from build123d import *

# Parameters (mm, degrees)
F0_W     = 70.4432
F0_H     = 95.6654
F0_R     = 27.5
F1_DEPTH = 25
F2_R     = 5.08


with BuildPart() as f1:
    # F0 (on Top) → F1 (new body)
    with BuildSketch(Plane.XY):
        with Locations((0, -15.2273)):
            Rectangle(F0_W, F0_H)
        Circle(F0_R, mode=Mode.SUBTRACT)
    extrude(amount=F1_DEPTH)

    # F2
    f2_edges = [f1.edges().sort_by_distance(p)[0] for p in [
        (35.2216, -15.2273, 25),
        (35.2216, -15.2273, 0),
        (-35.2216, -15.2273, 25),
        (-35.2216, -15.2273, 0),
        (-35.2216, 32.6054, 12.5),
        (35.2216, 32.6054, 12.5),
        (0, 32.6054, 25),
        (0, 32.6054, 0),
    ]]
    fillet(f2_edges, radius=F2_R)


solid = f1.part
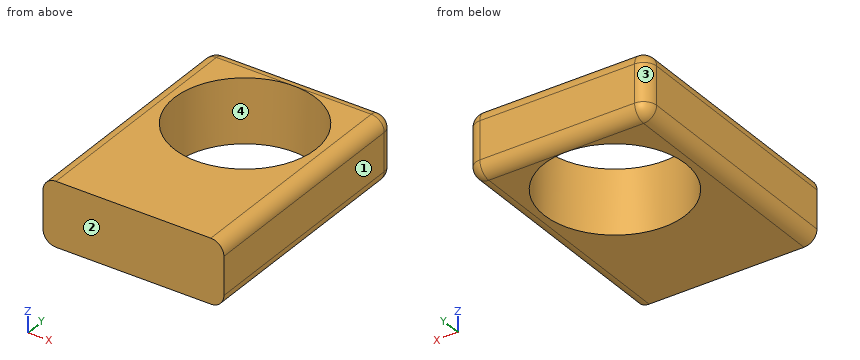
Geometry check sheet. Reference: the model listing, model coordinates, mm. Face numbers are marked on the shaded views. Round coordinates to 2 decimals unless told otherwise and drop trailing zeros. Order: outer loops, then holes, each group sorted by start corner. A loop starts at its lowest first (then second) coordinate and runs counter-clockwise, first axis right, second up. Notation, with made-up numbers: (14.25, -34.5) - (45.25, -34.5) arc R23 ccw to (45.25, -0.5) - close; hole circle Ø2 at (-4.75, 85.25). An arc over 180 degrees is marked (long way). One line per question, with ' | ' between items. Start each with the question number.
(1) Release check for a two-part mould opening along Y. For the marked faces 1, 2, 3 and 4 record: released by +Y, released by -Y, zero draft, split by the parting line, or undercut.
(2) Sectioned sample at C-C on z = 13.5. Record the cut outline in (x, y), and give its area (3 significant figures).
(3) Thickness scan on L1, parallel to Y at x = 0, z = 9.5; L2, parallel to X at y = 7.5, z = 3.25; L3, parallel to Y at x = -12, z = 4.25. Record the ranges inside material, lowest first. Write a range as [from, to].
(4) Sectioned sample at A-A on y = 0. Record the cut outline in (x, z).
(5) Sectioned sample at D-D on x = 17.5. Record the cut outline in (y, z).
Conclusion:
1) face 1: zero draft | face 2: released by -Y | face 3: released by +Y | face 4: undercut
2) outline: (-35.22, -63.06) - (35.22, -63.06) - (35.22, 27.53) arc R5.08 ccw to (30.14, 32.61) - (-30.14, 32.61) arc R5.08 ccw to (-35.22, 27.53) - close; hole circle Ø55 at (0, 0) | area: 4,350 mm2
3) L1: y = [-63.06, -27.5], [27.5, 32.61] | L2: x = [-34.88, -26.46], [26.46, 34.88] | L3: y = [-63.06, -24.74], [24.74, 32.54]
4) outline: (-35.22, 5.08) arc R5.08 ccw to (-30.14, 0) - (-27.5, 0) - (-27.5, 25) - (-30.14, 25) arc R5.08 ccw to (-35.22, 19.92) - close; (27.5, 0) - (30.14, 0) arc R5.08 ccw to (35.22, 5.08) - (35.22, 19.92) arc R5.08 ccw to (30.14, 25) - (27.5, 25) - close
5) outline: (-63.06, 0) - (-21.21, 0) - (-21.21, 25) - (-63.06, 25) - close; (21.21, 0) - (27.53, 0) arc R5.08 ccw to (32.61, 5.08) - (32.61, 19.92) arc R5.08 ccw to (27.53, 25) - (21.21, 25) - close
